Source: CAD feature listing. Evaluate the final solid. Frame: model axes, mm. A direction names the side the tool comes from. Coordinates: 2 decimals unless noted, no trailing zeros. Order: outer loops, then holes, each group sorted by start corner. A loop starts at its lowest first (then second) coordinate and runs counter-clockwise, first axis right, second up.
```python
from build123d import *

# Parameters (mm, degrees)
SKETCH_1_W               = 59.4
SKETCH_1_H               = 43.4
EXTRUDE_1_DEPTH          = 6
SKETCH_2_W               = 56.4
SKETCH_2_H               = 40.4
CUT_EXTRUDE_1_DEPTH      = 4.5
SKETCH_3_R               = 1.25
CUT_EXTRUDE_2_DEPTH      = 2.5
SKETCH_4_W               = 10.95
SKETCH_4_H               = 10.5
CUT_EXTRUDE_3_DEPTH      = 5.5
CUT_EXTRUDE_3_DEPTH_BACK = 2.5
SKETCH_5_W               = 6.4
SKETCH_5_H               = 4.5
SKETCH_5_W_2             = 6.3
CUT_EXTRUDE_4_DEPTH      = 4.5
CUT_EXTRUDE_5_DEPTH      = 5.5
CUT_EXTRUDE_5_DEPTH_BACK = 2.5
SKETCH_9_W               = 10.2
SKETCH_9_H               = 8.8
SKETCH_9_W_2             = 4.7
CUT_EXTRUDE_6_DEPTH      = 5.5
CUT_EXTRUDE_6_DEPTH_BACK = 2.5
SKETCH_10_W              = 8
SKETCH_10_H              = 13.3
CUT_EXTRUDE_7_DEPTH      = 5.5
CUT_EXTRUDE_7_DEPTH_BACK = 2.5
FILLET_1_R               = 2
SKETCH_11_W              = 8.5
SKETCH_11_H              = 4.5
SKETCH_11_W_2            = 18
CUT_EXTRUDE_8_DEPTH      = 3
SKETCH_12_W              = 9.25
SKETCH_12_H              = 4.5
SKETCH_12_W_2            = 21
CUT_EXTRUDE_9_DEPTH      = 3
SKETCH_13_W              = 16.5
SKETCH_13_H              = 4.5
CUT_EXTRUDE_10_DEPTH     = 3
SKETCH_14_W              = 7.5
SKETCH_14_H              = 13.2
CUT_EXTRUDE_11_DEPTH     = 10
FILLET_2_R               = 0.5
FILLET_3_R               = 1
FILLET_4_R               = 0.5


with BuildPart() as part:
    # 草图1 → 凸台-拉伸1 (new body)
    with BuildSketch(Plane(origin=(0, 0, 0), x_dir=(1, 0, 0), z_dir=(0, 1, 0))):
        Rectangle(SKETCH_1_W, SKETCH_1_H)
    extrude(amount=EXTRUDE_1_DEPTH)

    # 草图2 → 切除-拉伸1 (cut)
    with BuildSketch(Plane(origin=(0, 6, 0), x_dir=(1, 0, 0), z_dir=(0, 1, 0))):
        Rectangle(SKETCH_2_W, SKETCH_2_H)
    extrude(amount=-CUT_EXTRUDE_1_DEPTH, mode=Mode.SUBTRACT)

    # 草图3 → 切除-拉伸2 (cut, through all)
    with BuildSketch(Plane(origin=(0, 1.5, 0), x_dir=(1, 0, 0), z_dir=(0, 1, 0))):
        with Locations((-10.2, -18)):
            Circle(SKETCH_3_R)
        with Locations((-10.2, 18)):
            Circle(SKETCH_3_R)
        with Locations((25.8, 18)):
            Circle(SKETCH_3_R)
        with Locations((25.8, -18)):
            Circle(SKETCH_3_R)
    extrude(amount=-CUT_EXTRUDE_2_DEPTH, mode=Mode.SUBTRACT)

    # 草图4 → 切除-拉伸3 (cut, two sides)
    with BuildSketch(Plane(origin=(0, 1.5, 0), x_dir=(1, 0, 0), z_dir=(0, 1, 0))) as cut_extrude_3_sk:
        with Locations((-24.225, -0.05)):
            Rectangle(SKETCH_4_W, SKETCH_4_H)
    extrude(amount=CUT_EXTRUDE_3_DEPTH, mode=Mode.SUBTRACT)
    extrude(cut_extrude_3_sk.sketch, amount=-CUT_EXTRUDE_3_DEPTH_BACK, mode=Mode.SUBTRACT)

    # 草图5 → 切除-拉伸4 (cut)
    with BuildSketch(Plane.ZY.offset(29.7)):
        with Locations((-9.8, 3.75)):
            Rectangle(SKETCH_5_W, SKETCH_5_H)
        with Locations((9.85, 3.75)):
            Rectangle(SKETCH_5_W_2, SKETCH_5_H)
    extrude(amount=-CUT_EXTRUDE_4_DEPTH, mode=Mode.SUBTRACT)

    # 草图8 → 切除-拉伸5 (cut, two sides)
    with BuildSketch(Plane(origin=(0, 1.5, 0), x_dir=(1, 0, 0), z_dir=(0, 1, 0))) as cut_extrude_5_sk:
        Polygon((-28.05, 14.35), (-28.05, 16.6), (-28.45, 16.6), (-28.45, 17.8), (-28.05, 17.8), (-28.05, 20.05), (-12.75, 20.05), (-12.75, 17.8), (-12.35, 17.8), (-12.35, 16.6), (-12.75, 16.6), (-12.75, 14.35), align=None)
        Polygon((-28.05, -20.05), (-12.75, -20.05), (-12.75, -17.8), (-12.35, -17.8), (-12.35, -16.6), (-12.75, -16.6), (-12.75, -14.35), (-28.05, -14.35), (-28.05, -16.6), (-28.45, -16.6), (-28.45, -17.8), (-28.05, -17.8), align=None)
    extrude(amount=CUT_EXTRUDE_5_DEPTH, mode=Mode.SUBTRACT)
    extrude(cut_extrude_5_sk.sketch, amount=-CUT_EXTRUDE_5_DEPTH_BACK, mode=Mode.SUBTRACT)

    # 草图9 → 切除-拉伸6 (cut, two sides)
    with BuildSketch(Plane(origin=(0, 1.5, 0), x_dir=(1, 0, 0), z_dir=(0, 1, 0))) as cut_extrude_6_sk:
        with Locations((-7.2, 11)):
            Rectangle(SKETCH_9_W, SKETCH_9_H)
        with Locations((-9.95, -11)):
            Rectangle(SKETCH_9_W_2, SKETCH_9_H)
    extrude(amount=CUT_EXTRUDE_6_DEPTH, mode=Mode.SUBTRACT)
    extrude(cut_extrude_6_sk.sketch, amount=-CUT_EXTRUDE_6_DEPTH_BACK, mode=Mode.SUBTRACT)

    # 草图10 → 切除-拉伸7 (cut, two sides)
    with BuildSketch(Plane(origin=(0, 1.5, 0), x_dir=(1, 0, 0), z_dir=(0, 1, 0))) as cut_extrude_7_sk:
        with Locations((24.05, -7.55)):
            Rectangle(SKETCH_10_W, SKETCH_10_H)
    extrude(amount=CUT_EXTRUDE_7_DEPTH, mode=Mode.SUBTRACT)
    extrude(cut_extrude_7_sk.sketch, amount=-CUT_EXTRUDE_7_DEPTH_BACK, mode=Mode.SUBTRACT)

    # 圆角1
    fillet_1_edges = [part.edges().sort_by_distance(p)[0] for p in [
        (29.7, 3, 21.7),
        (-29.7, 3, 21.7),
        (-29.7, 3, -21.7),
        (29.7, 3, -21.7),
    ]]
    fillet(fillet_1_edges, radius=FILLET_1_R)

    # 草图11 → 切除-拉伸8 (cut)
    with BuildSketch(Plane(origin=(0, 0, -21.7), x_dir=(-1, 0, 0), z_dir=(0, 0, -1))):
        with Locations((4.75, 3.75)):
            Rectangle(SKETCH_11_W, SKETCH_11_H)
        with Locations((-14.5, 3.75)):
            Rectangle(SKETCH_11_W_2, SKETCH_11_H)
    extrude(amount=-CUT_EXTRUDE_8_DEPTH, mode=Mode.SUBTRACT)

    # 草图12 → 切除-拉伸9 (cut)
    with BuildSketch(Plane.XY.offset(21.7)):
        with Locations((-2.875, 3.75)):
            Rectangle(SKETCH_12_W, SKETCH_12_H)
        with Locations((13, 3.75)):
            Rectangle(SKETCH_12_W_2, SKETCH_12_H)
    extrude(amount=-CUT_EXTRUDE_9_DEPTH, mode=Mode.SUBTRACT)

    # 草图13 → 切除-拉伸10 (cut)
    with BuildSketch(Plane(origin=(29.7, 0, 0), x_dir=(0, 0, -1), z_dir=(1, 0, 0))):
        with Locations((7.25, 3.75)):
            Rectangle(SKETCH_13_W, SKETCH_13_H)
    extrude(amount=-CUT_EXTRUDE_10_DEPTH, mode=Mode.SUBTRACT)

    # 草图14 → 切除-拉伸11 (cut)
    with BuildSketch(Plane.XZ):
        with Locations((-3.35, 0)):
            Rectangle(SKETCH_14_W, SKETCH_14_H)
    extrude(amount=-CUT_EXTRUDE_11_DEPTH, mode=Mode.SUBTRACT)

    # 圆角2
    fillet_2_edges = [part.edges().sort_by_distance(p)[0] for p in [
        (-12.3, 0.75, -15.4),
        (-2.1, 0.75, -15.4),
        (-2.1, 0.75, -6.6),
        (-12.3, 0.75, -6.6),
        (-12.3, 0.75, 15.4),
        (-12.3, 0.75, 6.6),
        (-7.6, 0.75, 6.6),
        (-7.6, 0.75, 15.4),
        (28.05, 0.75, 0.9),
        (28.05, 0.75, 14.2),
        (20.05, 0.75, 14.2),
        (20.05, 0.75, 0.9),
        (-7.1, 0.75, -6.6),
        (0.4, 0.75, -6.6),
        (0.4, 0.75, 6.6),
        (-7.1, 0.75, 6.6),
        (-18.75, 0.75, 5.3),
        (-18.75, 0.75, -5.2),
    ]]
    fillet(fillet_2_edges, radius=FILLET_2_R)

    # 圆角3
    fillet_3_edges = [part.edges().sort_by_distance(p)[0] for p in [
        (-28.05, 0.75, 14.35),
        (-12.75, 0.75, 14.35),
        (-12.75, 0.75, 20.05),
        (-28.05, 0.75, 20.05),
        (28.2, 3.75, -20.2),
        (-12.75, 0.75, -20.05),
        (-12.75, 0.75, -14.35),
        (-28.05, 0.75, -14.35),
        (-28.05, 0.75, -20.05),
        (-28.2, 3.75, 20.2),
        (-28.2, 3.75, -20.2),
    ]]
    fillet(fillet_3_edges, radius=FILLET_3_R)

    # 圆角4
    fillet_4_edges = [part.edges().sort_by_distance(p)[0] for p in [
        (23.5, 1.5, -20.95),
        (-9, 1.5, -20.95),
        (-0.5, 1.5, -20.95),
        (23.5, 1.5, 20.95),
        (2.5, 1.5, 20.95),
        (1.75, 1.5, 20.95),
        (-7.5, 1.5, 20.95),
        (28.95, 1.5, 1),
        (28.95, 1.5, -15.5),
        (-28.95, 1.5, -6.6),
        (-28.95, 1.5, -13),
        (-28.95, 1.5, 13),
        (-28.95, 1.5, 6.7),
    ]]
    fillet(fillet_4_edges, radius=FILLET_4_R)


solid = part.part
```
1. Pin query (flat end, axial travel): P1, Ø0.8, axis at x = -29, y = 5, coming from the -Z side; P2, Ø10, axis at x = 3.5, z = 7, coming from the -Y side; P3, Ø4, axis at x = -13.5, z = -14.5, coming from the +Y side. Return the tip coordinate at first contact, or that it passes through.
Findings:
P1: stops at z = -21.49
P2: stops at y = 0
P3: stops at y = 1.5
2. Access query for faces 1 (the face through (23.5, 4, 21)), 2 (the face through (-28.2, 4, -15)), 3 (the face through (-29, 4, 6.7)), 4 (the face through (-12.35, 1, 17)). Directions: +Z, -Z, +X, -X, +Y, -Y. A direction counts if a zero-diameter tool reaches every point of the face in a straight line with its end or side. Return the directions, or none.
Findings:
face 1: +Z, -Z, +Y
face 2: +Y
face 3: -X, +Y
face 4: +Y, -Y
3. Section query C-C on x = -14.5. Return loops of the section in (y, z), plus the area to 3 significant figures.
Findings:
outline: (0, -21.7) - (6, -21.7) - (6, -20.2) - (1.5, -20.2) - (1.5, -20.05) - (0, -20.05) - close; (0, -14.35) - (1.5, -14.35) - (1.5, 14.35) - (0, 14.35) - close; (0, 20.05) - (1.5, 20.05) - (1.5, 20.2) - (6, 20.2) - (6, 21.7) - (0, 21.7) - close
area: 61.5 mm2
4. Section query A-A on x = -24.5. Return loops of the section in (y, z).
Findings:
outline: (0, -21.7) - (6, -21.7) - (6, -20.2) - (1.5, -20.2) - (1.5, -20.05) - (0, -20.05) - close; (0, -14.35) - (1.5, -14.35) - (1.5, -5.2) - (0, -5.2) - close; (0, 5.3) - (1.5, 5.3) - (1.5, 14.35) - (0, 14.35) - close; (0, 20.05) - (1.5, 20.05) - (1.5, 20.2) - (6, 20.2) - (6, 21.7) - (0, 21.7) - close
5. Draft query along X for faces 5 (the face through (29.13, 3.04, -21.1)), 6 (the face through (28.05, 1, 8)), 7 (the face through (-7, 1, 21.7)). Return one class per face: released by +X, released by -X, zero draft, split by the parting line, or undercut.
Findings:
face 5: released by +X
face 6: undercut
face 7: zero draft
6. Ray query, line 1 (Z direction, x = -10.2, y = 0.9); line 2 (X direction, y = 0.4, z = -18); line 3 (Z direction, x = 25, y = 5.4). Return the intervals inside material, ascending.
Findings:
line 1: z = -21.7 to -19.25, -16.75 to -15.4, -6.6 to 6.6, 15.4 to 16.75, 19.25 to 21.7
line 2: x = -29.7 to -28.05, -12.75 to -11.45, -8.95 to 24.55, 27.05 to 29.7
line 3: z = -21.7 to -20.2, 20.2 to 21.7
7. Section query B-B on z = -4. Return loops of the section in (x, y), plus the area to 3 significant figures.
Findings:
outline: (-18.75, 0) - (-7.1, 0) - (-7.1, 1.5) - (-18.75, 1.5) - close; (0.4, 0) - (29.7, 0) - (29.7, 1.5) - (0.4, 1.5) - close
area: 61.4 mm2
8. Section query D-D on y = 4.95. Count the separate pieces of the cut face and the enclosed holes in it, plus the area to 3 significant figures.
Findings:
separate pieces: 8
enclosed holes: 0
area: 151 mm2
